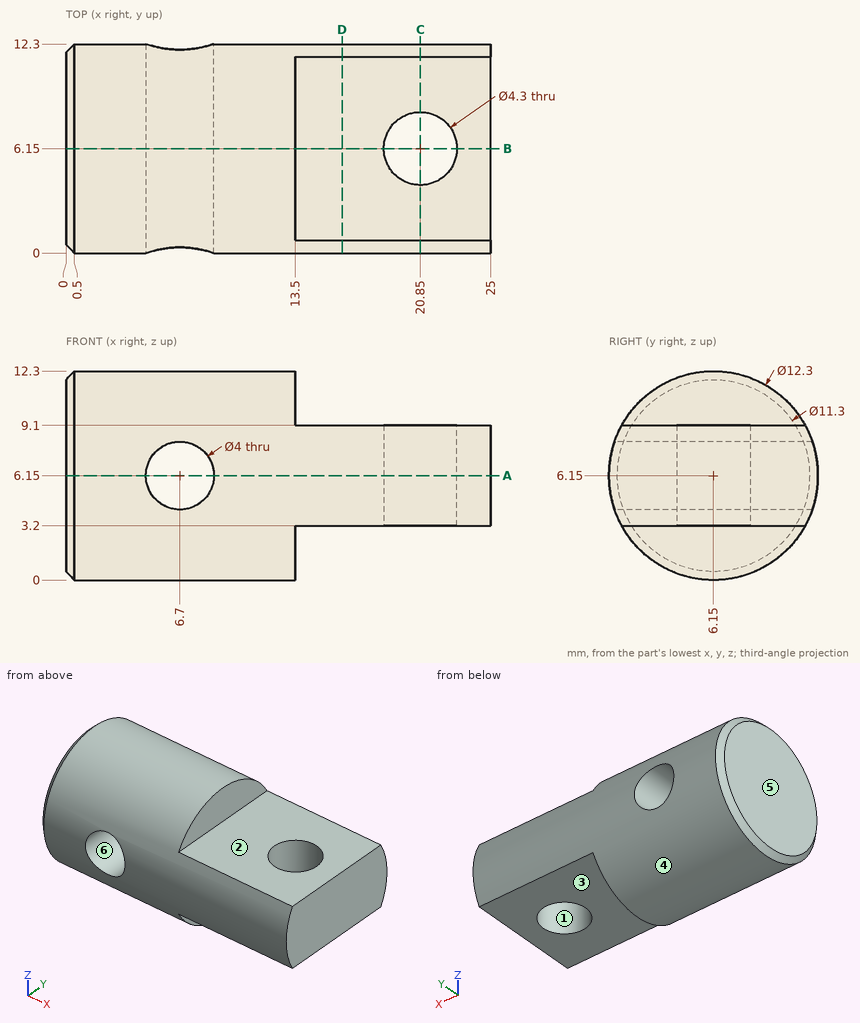
Can you work these out from the drawing? Everything is in mm from the part's minimum corner. A direction names the side the tool comes from. Give positions to 0.01 mm unless a question says otherwise; leave off trailing zeros. Order: outer loops, then holes, each group sorted by start corner. A loop starts at its lowest first (then second) coordinate and runs counter-clockwise, first axis right, second up.
Item 1: For the marked faces 1 and 2, which set-ups out of +Z, -Z, +X, -X, +Y, -Y let a thin tool reach every point of the face, with its end or its side?
Item 2: If we section it at A-A, the plane z = 6.15: Write out the boundary of the cut face in (x, y).
Item 3: I'm going to push flat-ended pins straight in: pin 1 (5 mm diameter, centred on x = 20.85, y = 6.15, fed in from +Z); pin 2 (6 mm diameter, centred on x = 17, z = 11, fed in from -Y); pin 3 (3.5 mm diameter, centred on y = 5, z = 11.5, fed in from +X). Where does each tip first touch, or does it pass through?
Item 4: If we section it at B-B, the plane y = 6.15: Write out the boundary of the cut face in (x, z), plus the area to 3 significant figures.
Item 5: I need wall thicknesses on line 1 (X direction, y = 3.25, z = 6); line 2 (Z direction, x = 6.7, y = 4.75); line 3 (X direction, y = 6.75, z = 4). Which ranges of each line are inside material? Lowest first, please.
Item 6: If we mould it in two halves opening along Z, with no side actions, what happens to the marked faces 3, 4, 5 and 6? For each: pulls with the +Z half, pulls with the -Z half, needs draft (parallel to the pull), parting line crosses it, or undercut.
Item 7: If we section it at D-D, the plane x = 16.25: Write out the boundary of the cut face in (y, z).
Item 8: If we section it at C-C, the plane x = 20.85: Write out the boundary of the cut face in (y, z).
Values:
1. face 1: +Z, -Z
1. face 2: +Z, +X, +Y, -Y
2. outline: (0, 0.5) - (0.5, 0) - (4.7, 0) - (4.7, 12.3) - (0.5, 12.3) - (0, 11.8) - close; (8.7, 0) - (25, 0) - (25, 12.3) - (8.7, 12.3) - close; hole circle Ø4.3 at (20.85, 6.15)
3. pin 1: stops at z = 9.1
3. pin 2: stops at y = 0.28
3. pin 3: stops at x = 13.5
4. outline: (0, 0.5) - (0.5, 0) - (13.5, 0) - (13.5, 3.2) - (18.7, 3.2) - (18.7, 9.1) - (13.5, 9.1) - (13.5, 12.3) - (0.5, 12.3) - (0, 11.8) - close; (23, 3.2) - (25, 3.2) - (25, 9.1) - (23, 9.1) - close; hole circle Ø4 at (6.7, 6.15)
4. area: 196 mm2
5. line 1: x = 0 to 4.71, 8.69 to 25
5. line 2: z = 0.16 to 4.15, 8.15 to 12.14
5. line 3: x = 0 to 18.79, 22.91 to 25
6. face 3: pulls with the -Z half
6. face 4: parting line crosses it
6. face 5: needs draft
6. face 6: undercut
7. outline: (0.75, 3.2) - (11.55, 3.2) arc R6.15 ccw to (11.55, 9.1) - (0.75, 9.1) arc R6.15 ccw to start
8. outline: (0.75, 3.2) - (4, 3.2) - (4, 9.1) - (0.75, 9.1) arc R6.15 ccw to start; (8.3, 3.2) - (11.55, 3.2) arc R6.15 ccw to (11.55, 9.1) - (8.3, 9.1) - close
